CAD build for the part. Positions are in the model's coordinates, mm. Give positions to 0.01 mm unless a question says otherwise; leave off trailing zeros. Answer as CSV lines item,"result".
```python
from build123d import *

# Parameters (mm, degrees)
SKETCH1_R           = 3.4036
BOSS_EXTRUDE1_DEPTH = 457.2


with BuildPart() as part:
    # Sketch1 → Boss-Extrude1 (new body, symmetric)
    with BuildSketch(Plane.XY):
        with BuildLine():
            Line((-39.878, 16.891), (-39.878, 4.7625))
            ThreePointArc((-39.878, 4.7625), (-39.654815367, 4.223684633), (-39.116, 4.0005))
            Line((-39.116, 4.0005), (-36.1442, 4.0005))
            ThreePointArc((-36.1442, 4.0005), (-35.605384633, 4.223684633), (-35.3822, 4.7625))
            Line((-35.3822, 4.7625), (-35.3822, 10.2235))
            ThreePointArc((-35.3822, 10.2235), (-34.911804775, 10.927496204), (-34.081384633, 10.762315367))
            Line((-34.081384633, 10.762315367), (-28.513059555, 5.19399029))
            ThreePointArc((-28.513059555, 5.19399029), (-27.863348265, 4.221628629), (-27.6352, 3.074649845))
            Line((-27.6352, 3.074649845), (-27.6352, -3.074649845))
            ThreePointArc((-27.6352, -3.074649845), (-27.863348265, -4.221628629), (-28.513059555, -5.19399029))
            Line((-28.513059555, -5.19399029), (-34.081384633, -10.762315367))
            ThreePointArc((-34.081384633, -10.762315367), (-34.911804775, -10.927496204), (-35.3822, -10.2235))
            Line((-35.3822, -10.2235), (-35.3822, -4.7625))
            ThreePointArc((-35.3822, -4.7625), (-35.605384633, -4.223684633), (-36.1442, -4.0005))
            Line((-36.1442, -4.0005), (-39.116, -4.0005))
            ThreePointArc((-39.116, -4.0005), (-39.654815367, -4.223684633), (-39.878, -4.7625))
            Line((-39.878, -4.7625), (-39.878, -16.891))
            ThreePointArc((-39.878, -16.891), (-38.985261469, -19.046261469), (-36.83, -19.939))
            Line((-36.83, -19.939), (-24.7015, -19.939))
            ThreePointArc((-24.7015, -19.939), (-24.162684633, -19.715815367), (-23.9395, -19.177))
            Line((-23.9395, -19.177), (-23.9395, -16.2052))
            ThreePointArc((-23.9395, -16.2052), (-24.162684633, -15.666384633), (-24.7015, -15.4432))
            Line((-24.7015, -15.4432), (-30.1625, -15.4432))
            ThreePointArc((-30.1625, -15.4432), (-30.866496204, -14.972804775), (-30.701315367, -14.142384633))
            Line((-30.701315367, -14.142384633), (-25.13299029, -8.574059555))
            ThreePointArc((-25.13299029, -8.574059555), (-24.160628629, -7.924348265), (-23.013649845, -7.6962))
            Line((-23.013649845, -7.6962), (-16.864350155, -7.6962))
            ThreePointArc((-16.864350155, -7.6962), (-15.717371371, -7.924348265), (-14.74500971, -8.574059555))
            Line((-14.74500971, -8.574059555), (-9.176684633, -14.142384633))
            ThreePointArc((-9.176684633, -14.142384633), (-9.011503796, -14.972804775), (-9.7155, -15.4432))
            Line((-9.7155, -15.4432), (-15.1765, -15.4432))
            ThreePointArc((-15.1765, -15.4432), (-15.715315367, -15.666384633), (-15.9385, -16.2052))
            Line((-15.9385, -16.2052), (-15.9385, -19.177))
            ThreePointArc((-15.9385, -19.177), (-15.715315367, -19.715815367), (-15.1765, -19.939))
            Line((-15.1765, -19.939), (15.1765, -19.939))
            ThreePointArc((15.1765, -19.939), (15.715315367, -19.715815367), (15.9385, -19.177))
            Line((15.9385, -19.177), (15.9385, -16.2052))
            ThreePointArc((15.9385, -16.2052), (15.715315367, -15.666384633), (15.1765, -15.4432))
            Line((15.1765, -15.4432), (9.7155, -15.4432))
            ThreePointArc((9.7155, -15.4432), (9.011503796, -14.972804775), (9.176684633, -14.142384633))
            Line((9.176684633, -14.142384633), (14.74500971, -8.574059555))
            ThreePointArc((14.74500971, -8.574059555), (15.717371371, -7.924348265), (16.864350155, -7.6962))
            Line((16.864350155, -7.6962), (23.013649845, -7.6962))
            ThreePointArc((23.013649845, -7.6962), (24.160628629, -7.924348265), (25.13299029, -8.574059555))
            Line((25.13299029, -8.574059555), (30.701315367, -14.142384633))
            ThreePointArc((30.701315367, -14.142384633), (30.866496204, -14.972804775), (30.1625, -15.4432))
            Line((30.1625, -15.4432), (24.7015, -15.4432))
            ThreePointArc((24.7015, -15.4432), (24.162684633, -15.666384633), (23.9395, -16.2052))
            Line((23.9395, -16.2052), (23.9395, -19.177))
            ThreePointArc((23.9395, -19.177), (24.162684633, -19.715815367), (24.7015, -19.939))
            Line((24.7015, -19.939), (36.83, -19.939))
            ThreePointArc((36.83, -19.939), (38.985261469, -19.046261469), (39.878, -16.891))
            Line((39.878, -16.891), (39.878, -4.7625))
            ThreePointArc((39.878, -4.7625), (39.654815367, -4.223684633), (39.116, -4.0005))
            Line((39.116, -4.0005), (36.1442, -4.0005))
            ThreePointArc((36.1442, -4.0005), (35.605384633, -4.223684633), (35.3822, -4.7625))
            Line((35.3822, -4.7625), (35.3822, -10.2235))
            ThreePointArc((35.3822, -10.2235), (34.911804775, -10.927496204), (34.081384633, -10.762315367))
            Line((34.081384633, -10.762315367), (28.513059555, -5.19399029))
            ThreePointArc((28.513059555, -5.19399029), (27.863348265, -4.221628629), (27.6352, -3.074649845))
            Line((27.6352, -3.074649845), (27.6352, 3.074649845))
            ThreePointArc((27.6352, 3.074649845), (27.863348265, 4.221628629), (28.513059555, 5.19399029))
            Line((28.513059555, 5.19399029), (34.081384633, 10.762315367))
            ThreePointArc((34.081384633, 10.762315367), (34.911804775, 10.927496204), (35.3822, 10.2235))
            Line((35.3822, 10.2235), (35.3822, 4.7625))
            ThreePointArc((35.3822, 4.7625), (35.605384633, 4.223684633), (36.1442, 4.0005))
            Line((36.1442, 4.0005), (39.116, 4.0005))
            ThreePointArc((39.116, 4.0005), (39.654815367, 4.223684633), (39.878, 4.7625))
            Line((39.878, 4.7625), (39.878, 16.891))
            ThreePointArc((39.878, 16.891), (38.985261469, 19.046261469), (36.83, 19.939))
            Line((36.83, 19.939), (24.7015, 19.939))
            ThreePointArc((24.7015, 19.939), (24.162684633, 19.715815367), (23.9395, 19.177))
            Line((23.9395, 19.177), (23.9395, 16.2052))
            ThreePointArc((23.9395, 16.2052), (24.162684633, 15.666384633), (24.7015, 15.4432))
            Line((24.7015, 15.4432), (30.1625, 15.4432))
            ThreePointArc((30.1625, 15.4432), (30.866496204, 14.972804775), (30.701315367, 14.142384633))
            Line((30.701315367, 14.142384633), (25.13299029, 8.574059555))
            ThreePointArc((25.13299029, 8.574059555), (24.160628629, 7.924348265), (23.013649845, 7.6962))
            Line((23.013649845, 7.6962), (16.864350155, 7.6962))
            ThreePointArc((16.864350155, 7.6962), (15.717371371, 7.924348265), (14.74500971, 8.574059555))
            Line((14.74500971, 8.574059555), (9.176684633, 14.142384633))
            ThreePointArc((9.176684633, 14.142384633), (9.011503796, 14.972804775), (9.7155, 15.4432))
            Line((9.7155, 15.4432), (15.1765, 15.4432))
            ThreePointArc((15.1765, 15.4432), (15.715315367, 15.666384633), (15.9385, 16.2052))
            Line((15.9385, 16.2052), (15.9385, 19.177))
            ThreePointArc((15.9385, 19.177), (15.715315367, 19.715815367), (15.1765, 19.939))
            Line((15.1765, 19.939), (-15.1765, 19.939))
            ThreePointArc((-15.1765, 19.939), (-15.715315367, 19.715815367), (-15.9385, 19.177))
            Line((-15.9385, 19.177), (-15.9385, 16.2052))
            ThreePointArc((-15.9385, 16.2052), (-15.715315367, 15.666384633), (-15.1765, 15.4432))
            Line((-15.1765, 15.4432), (-9.7155, 15.4432))
            ThreePointArc((-9.7155, 15.4432), (-9.011503796, 14.972804775), (-9.176684633, 14.142384633))
            Line((-9.176684633, 14.142384633), (-14.74500971, 8.574059555))
            ThreePointArc((-14.74500971, 8.574059555), (-15.717371371, 7.924348265), (-16.864350155, 7.6962))
            Line((-16.864350155, 7.6962), (-23.013649845, 7.6962))
            ThreePointArc((-23.013649845, 7.6962), (-24.160628629, 7.924348265), (-25.13299029, 8.574059555))
            Line((-25.13299029, 8.574059555), (-30.701315367, 14.142384633))
            ThreePointArc((-30.701315367, 14.142384633), (-30.866496204, 14.972804775), (-30.1625, 15.4432))
            Line((-30.1625, 15.4432), (-24.7015, 15.4432))
            ThreePointArc((-24.7015, 15.4432), (-24.162684633, 15.666384633), (-23.9395, 16.2052))
            Line((-23.9395, 16.2052), (-23.9395, 19.177))
            ThreePointArc((-23.9395, 19.177), (-24.162684633, 19.715815367), (-24.7015, 19.939))
            Line((-24.7015, 19.939), (-36.83, 19.939))
            ThreePointArc((-36.83, 19.939), (-38.985261469, 19.046261469), (-39.878, 16.891))
        make_face()
        with Locations((-19.939, 0)):
            Circle(SKETCH1_R, mode=Mode.SUBTRACT)
        with Locations((19.939, 0)):
            Circle(SKETCH1_R, mode=Mode.SUBTRACT)
        with BuildLine():
            Line((-12.2428, 3.074649845), (-12.2428, -3.074649845))
            ThreePointArc((-12.2428, -3.074649845), (-12.014651735, -4.221628629), (-11.364940445, -5.19399029))
            Line((-11.364940445, -5.19399029), (-1.904671503, -14.654259232))
            ThreePointArc((-1.904671503, -14.654259232), (0, -15.4432), (1.904671503, -14.654259232))
            Line((1.904671503, -14.654259232), (11.364940445, -5.19399029))
            ThreePointArc((11.364940445, -5.19399029), (12.014651735, -4.221628629), (12.2428, -3.074649845))
            Line((12.2428, -3.074649845), (12.2428, 3.074649845))
            ThreePointArc((12.2428, 3.074649845), (12.014651735, 4.221628629), (11.364940445, 5.19399029))
            Line((11.364940445, 5.19399029), (1.904671503, 14.654259232))
            ThreePointArc((1.904671503, 14.654259232), (0, 15.4432), (-1.904671503, 14.654259232))
            Line((-1.904671503, 14.654259232), (-11.364940445, 5.19399029))
            ThreePointArc((-11.364940445, 5.19399029), (-12.014651735, 4.221628629), (-12.2428, 3.074649845))
        make_face(mode=Mode.SUBTRACT)
    extrude(amount=BOSS_EXTRUDE1_DEPTH, both=True)


solid = part.part
```
1) Band-saw the part on A-A, the plane z = 258.5. Give the number of separate pieces and of enclosed holes in the cut face, then the cut area to 3 significant figures.
Data:
separate pieces,"1"
enclosed holes,"3"
area,"1,620 mm2"
2) Pin check, flat tips, straight feed: P1, Ø0.9, axis at x = -38, z = -31, coming from the -Y side; P2, Ø5, axis at x = -19.5, z = -194.5, coming from the -Y side; P3, Ø1, axis at x = 16.5, z = 53, coming from the -Y side. Stop position of each tip, or through.
Data:
P1,"stops at y = -19.85"
P2,"stops at y = -7.7"
P3,"stops at y = -7.82"
3) Wall check: line 1 along X through (y, z) = (1.5, -128); line 2 along X through (y, z) = (17, 30.5); line 3 along Y through (x, z) = (-25, -256). Give the ranges that are in metal, low to high. Write a range as [from, to].
Data:
line 1,"x = [-27.64, -22.99], [-16.88, -12.24], [12.24, 16.88], [22.99, 27.64]"
line 2,"x = [-39.88, -23.94], [-15.94, 15.94], [23.94, 39.88]"
line 3,"y = [-19.94, -15.44], [-8.45, 8.45], [15.44, 19.94]"
